```python
from build123d import *

# Parameters (mm, degrees)
EXTRUDE_1_DEPTH     = 13
EXTRUDE_2_DEPTH     = 3
EXTRUDE_3_DEPTH     = 1
CUT_EXTRUDE_1_DEPTH = 16
SKETCH_5_W          = 2
SKETCH_5_H          = 5
EXTRUDE_4_DEPTH     = 15
FILLET_1_R          = 2
SKETCH_6_W          = 1.000000004
SKETCH_6_H          = 5
SKETCH_6_W_2        = 0.999999996
SKETCH_6_W_3        = 1
EXTRUDE_5_DEPTH     = 9
SKETCH_7_W          = 2.859887346
SKETCH_7_H          = 6.332607693
SKETCH_7_W_2        = 2.383674024
SKETCH_7_H_2        = 6.268510199
SKETCH_7_W_3        = 2.540472095
SKETCH_7_H_3        = 6.351983774
EXTRUDE_7_DEPTH     = 1.5
SKETCH_8_R          = 1.317694444
CUT_EXTRUDE_2_DEPTH = 21.5
SKETCH_9_R          = 1.323361973
CUT_EXTRUDE_3_DEPTH = 3.5
FILLET_2_R          = 2
SKETCH_10_R         = 2
CUT_EXTRUDE_4_DEPTH = 3.5
SKETCH_11_R         = 2
CUT_EXTRUDE_5_DEPTH = 3.5
CHAMFER_1_SIZE      = 1


with BuildPart() as part:
    # Эскиз1 → Бобышка-Вытянуть1 (new body)
    with BuildSketch(Plane.XY):
        with BuildLine():
            Line((-24.03751348, 4.570186882), (-3.03751348, 4.570186882))
            ThreePointArc((-3.03751348, 4.570186882), (-0.916193137, 3.691507225), (-0.03751348, 1.570186882))
            Line((-0.03751348, 1.570186882), (-0.03751348, -9.429813118))
            Line((-0.03751348, -9.429813118), (-5.53751348, -14.429813118))
            Line((-5.53751348, -14.429813118), (-21.53751348, -14.429813118))
            Line((-21.53751348, -14.429813118), (-27.03751348, -9.429813118))
            Line((-27.03751348, -9.429813118), (-27.03751348, 1.570186882))
            ThreePointArc((-27.03751348, 1.570186882), (-26.158833824, 3.691507225), (-24.03751348, 4.570186882))
        make_face()
    extrude(amount=EXTRUDE_1_DEPTH)

    # Эскиз2 → Бобышка-Вытянуть2 (add)
    with BuildSketch(Plane.XY.offset(13)):
        with BuildLine():
            Line((-24.253629022, 6.070186882), (-2.821397929, 6.070186882))
            ThreePointArc((-2.821397929, 6.070186882), (-1.598940451, 5.87880838), (-0.493459013, 5.322985739))
            Line((-0.493459013, 5.322985739), (9.290425441, -1.679071989))
            ThreePointArc((9.290425441, -1.679071989), (10.962486488, -4.932373697), (9.289607579, -8.185254927))
            Line((9.289607579, -8.185254927), (-0.493722264, -15.183197119))
            ThreePointArc((-0.493722264, -15.183197119), (-1.598864627, -15.738588249), (-2.820843349, -15.929813118))
            Line((-2.820843349, -15.929813118), (-24.254183602, -15.929813118))
            ThreePointArc((-24.254183602, -15.929813118), (-25.476162332, -15.738588247), (-26.5813047, -15.183197109))
            Line((-26.5813047, -15.183197109), (-36.364634505, -8.185254887))
            ThreePointArc((-36.364634505, -8.185254887), (-38.037513448, -4.932373739), (-36.365452436, -1.679072079))
            Line((-36.365452436, -1.679072079), (-26.581567951, 5.322985729))
            ThreePointArc((-26.581567951, 5.322985729), (-25.476086508, 5.878808377), (-24.253629022, 6.070186882))
        make_face()
    extrude(amount=EXTRUDE_2_DEPTH)

    # Эскиз3 → Бобышка-Вытянуть3 (add)
    with BuildSketch(Plane.XY.offset(16)):
        with BuildLine():
            Line((-24.254183602, -15.929813118), (-2.820843349, -15.929813118))
            ThreePointArc((-2.820843349, -15.929813118), (0.007639796, -14.758184221), (1.179156647, -11.929654667))
            Line((1.179156647, -11.929654667), (1.178602071, 2.070186882))
            ThreePointArc((1.178602071, 2.070186882), (0.007029196, 4.898614007), (-2.821397929, 6.070186882))
            Line((-2.821397929, 6.070186882), (-24.253629022, 6.070186882))
            ThreePointArc((-24.253629022, 6.070186882), (-27.082056147, 4.898614007), (-28.253629022, 2.070186882))
            Line((-28.253629022, 2.070186882), (-28.254183602, -11.929813118))
            ThreePointArc((-28.254183602, -11.929813118), (-27.082610727, -14.758240243), (-24.254183602, -15.929813118))
        make_face()
    extrude(amount=EXTRUDE_3_DEPTH)

    # Эскиз4 → Вырез-Вытянуть1 (cut)
    with BuildSketch(Plane.XY.offset(17)):
        with BuildLine():
            Line((-24.537513476, 3.070186882), (-2.537513476, 3.070186882))
            ThreePointArc((-2.537513476, 3.070186882), (-1.476853304, 2.630847054), (-1.037513476, 1.570186882))
            Line((-1.037513476, 1.570186882), (-1.037513476, -8.208875847))
            ThreePointArc((-1.037513476, -8.208875847), (-1.185558621, -8.858658943), (-1.600470904, -9.380179061))
            Line((-1.600470904, -9.380179061), (-5.626642493, -12.601116332))
            ThreePointArc((-5.626642493, -12.601116332), (-6.067174653, -12.845255597), (-6.563685065, -12.929813118))
            Line((-6.563685065, -12.929813118), (-20.511341887, -12.929813118))
            ThreePointArc((-20.511341887, -12.929813118), (-21.007852299, -12.845255597), (-21.448384458, -12.601116332))
            Line((-21.448384458, -12.601116332), (-25.474556047, -9.380179061))
            ThreePointArc((-25.474556047, -9.380179061), (-25.88946833, -8.858658943), (-26.037513476, -8.208875847))
            Line((-26.037513476, -8.208875847), (-26.037513476, 1.570186882))
            ThreePointArc((-26.037513476, 1.570186882), (-25.598173647, 2.630847054), (-24.537513476, 3.070186882))
        make_face()
    extrude(amount=-CUT_EXTRUDE_1_DEPTH, mode=Mode.SUBTRACT)

    # Эскиз5 → Бобышка-Вытянуть4 (add)
    with BuildSketch(Plane.XY.offset(1)):
        with Locations((-21.537513476, -1.775325657)):
            Rectangle(SKETCH_5_W, SKETCH_5_H)
        with Locations((-13.537513476, -6.926056238)):
            Rectangle(SKETCH_5_W, SKETCH_5_H)
        with Locations((-5.537513476, -1.775325657)):
            Rectangle(SKETCH_5_W, SKETCH_5_H)
    extrude(amount=EXTRUDE_4_DEPTH)

    # Скругление1
    fillet_1_edges = [part.edges().sort_by_distance(p)[0] for p in [
        (-21.537513476, -4.275325657, 16),
        (-21.537513476, 0.724674343, 16),
        (-13.537513476, -9.426056238, 16),
        (-13.537513476, -4.426056238, 16),
        (-5.537513476, -4.275325657, 16),
        (-5.537513476, 0.724674343, 16),
    ]]
    fillet(fillet_1_edges, radius=FILLET_1_R)

    # Эскиз6 → Бобышка-Вытянуть5 (add)
    with BuildSketch(Plane(origin=(0, 0, 0), x_dir=(-1, 0, 0), z_dir=(0, 0, -1))):
        with Locations((5.037513478, -1.775325657)):
            Rectangle(SKETCH_6_W, SKETCH_6_H)
        with Locations((22.037513478, -1.775325657)):
            Rectangle(SKETCH_6_W_2, SKETCH_6_H)
        with Locations((13.628958145, -6.926056238)):
            Rectangle(SKETCH_6_W_3, SKETCH_6_H)
    extrude(amount=EXTRUDE_5_DEPTH)

    # Эскиз7 → Бобышка-Вытянуть7 (add)
    with BuildSketch(Plane(origin=(0, 0, 0), x_dir=(-1, 0, 0), z_dir=(0, 0, -1))):
        with Locations((5.059990277, -1.840113397)):
            Rectangle(SKETCH_7_W, SKETCH_7_H)
        with Locations((13.656892737, -6.928034415)):
            Rectangle(SKETCH_7_W_2, SKETCH_7_H_2)
        with Locations((22.046734018, -1.830425356)):
            Rectangle(SKETCH_7_W_3, SKETCH_7_H_3)
    extrude(amount=EXTRUDE_7_DEPTH)

    # Эскиз8 → Вырез-Вытянуть2 (cut)
    with BuildSketch(Plane(origin=(-4.537513476, 0, 0), x_dir=(0, 0, -1), z_dir=(1, 0, 0))):
        with Locations((6.23718035, -1.561929148)):
            Circle(SKETCH_8_R)
    extrude(amount=-CUT_EXTRUDE_2_DEPTH, mode=Mode.SUBTRACT)

    # Эскиз9 → Вырез-Вытянуть3 (cut)
    with BuildSketch(Plane(origin=(-13.128958145, 0, 0), x_dir=(0, 0, -1), z_dir=(1, 0, 0))):
        with Locations((6.266853337, -6.932739708)):
            Circle(SKETCH_9_R)
    extrude(amount=-CUT_EXTRUDE_3_DEPTH, mode=Mode.SUBTRACT)

    # Скругление2
    fillet_2_edges = [part.edges().sort_by_distance(p)[0] for p in [
        (-5.037513478, -4.275325657, -9),
        (-5.037513478, 0.724674343, -9),
        (-22.037513478, 0.724674343, -9),
        (-22.037513478, -4.275325657, -9),
        (-13.628958145, -9.426056238, -9),
        (-13.628958145, -4.426056238, -9),
    ]]
    fillet(fillet_2_edges, radius=FILLET_2_R)

    # Эскиз10 → Вырез-Вытянуть4 (cut)
    with BuildSketch(Plane.XY.offset(16)):
        with Locations((6.462486524, -4.931870875)):
            Circle(SKETCH_10_R)
    extrude(amount=-CUT_EXTRUDE_4_DEPTH, mode=Mode.SUBTRACT)

    # Эскиз11 → Вырез-Вытянуть5 (cut)
    with BuildSketch(Plane.XY.offset(16)):
        with Locations((-33.537513476, -4.931870875)):
            Circle(SKETCH_11_R)
    extrude(amount=-CUT_EXTRUDE_5_DEPTH, mode=Mode.SUBTRACT)

    # Фаска1
    chamfer_1_edges = [part.edges().sort_by_distance(p)[0] for p in [
        (4.462486524, -4.931870875, 16),
        (-35.537513476, -4.931870875, 16),
    ]]
    chamfer(chamfer_1_edges, length=CHAMFER_1_SIZE)


solid = part.part
```
Can you work these out from the model? Positions are in its coordinate system, mm. A direction names the side the tool comes from. Coordinates: 2 decimals unless noted, no trailing zeros. Write each loop counter-clockwise with the first axis right and the second up, starting at its lowest first coordinate (ties: lowest second). Pieces come first, ordered by that corner, then holes. Notation, with made-up numbers: (15, 89.25) - (56, 89.25) arc R22 ccw to (56, 127.25) - close; hole circle Ø11 at (-3, 44). An arc over 180 degrees is marked (long way). Return JSON: item names as keys, results as strings.
Q1. If we section it at C-C (x = -8): Please give me the cut outline in (y, z).
Computed values:
{"outline": "(-15.93, 13) - (-14.43, 13) - (-14.43, 0) - (4.57, 0) - (4.57, 13) - (6.07, 13) - (6.07, 17) - (3.07, 17) - (3.07, 1) - (-12.93, 1) - (-12.93, 17) - (-15.93, 17) - close"}
Q2. If we section it at A-A (z = 11.5): Count the separate pieces of the cut face and the enclosed holes in it, then the cut area to 3 significant figures.
Computed values:
{"separate pieces": "4", "enclosed holes": "1", "area": "133 mm2"}
Q3. If we section it at D-D (z = -5.5): Please give me the cut outline in (x, y).
Computed values:
{"outline": "(-22.54, -4.28) - (-21.54, -4.28) - (-21.54, -2.65) - (-22.54, -2.65) - close; (-22.54, -0.47) - (-21.54, -0.47) - (-21.54, 0.72) - (-22.54, 0.72) - close; (-14.13, -9.43) - (-13.13, -9.43) - (-13.13, -8.01) - (-14.13, -8.01) - close; (-14.13, -5.85) - (-13.13, -5.85) - (-13.13, -4.43) - (-14.13, -4.43) - close; (-5.54, -4.28) - (-4.54, -4.28) - (-4.54, -2.65) - (-5.54, -2.65) - close; (-5.54, -0.47) - (-4.54, -0.47) - (-4.54, 0.72) - (-5.54, 0.72) - close"}
Q4. Please list where these lines run through material, in increasing order: L1, parallel to X at y = -4.5, z = -1.25; L2, parallel to X at y = 0.5, z = -0.25; L3, parallel to X at y = -2.25, z = 10. Write a range as from..to.
Computed values:
{"L1": "x = -23.32..-20.78, -14.85..-12.47, -6.49..-3.63", "L2": "x = -23.32..-20.78, -6.49..-3.63", "L3": "x = -27.04..-26.04, -22.54..-20.54, -6.54..-4.54, -1.04..-0.04"}
Q5. I'm going to push flat-ended pins straight in: pin 1 Ø3 at (x, z) = (-15, 1.5) entering from -Y; pin 2 Ø10 at (y, z) = (-5, 1.5) entering from +X; pin 3 Ø1.6 at (x, z) = (-5.5, 4.5) entering from +Y. Where does each tip first touch, or does it pass through?
Computed values:
{"pin 1": "stops at y = -14.43", "pin 2": "stops at x = -0.04", "pin 3": "stops at y = 4.57"}
Q6. On a 3-axis mill with a long thin cutter (end or side, diameter ignored), from which of +Z, -Z, +X, -X, +Y, -Y can I reach the whole of each face in a straight line? I mean faces 4 (the flat face through (-13, -15, 13)), 5 (the flat face through (-22, -5.006, -1)), 6 (the cylindrical face through (-21.524, -3.705, 15.399)), 7 (the flat face through (-5.538, -2, -4)). Say none if no direction works.
Computed values:
{"face 4": "-Z", "face 5": "-Z, -X, -Y", "face 6": "+Z", "face 7": "-Z, +Y, -Y"}
Q7. Thinking about a two-plate mould opening in Y: for faces 1 (the flat face through (-31.542, 1.773, 14.479)), 2 (the flat face through (-4.538, -2, -4)), 3 (the flat face through (-22, -4.275, 7)), which applies, +Y half, -Y half, draft (parallel to the pull), parting line (faces both ways), or undercut?
Computed values:
{"face 1": "+Y half", "face 2": "draft", "face 3": "undercut"}
Q8. If we section it at B-B (z = -0.5): Please give me the cut outline in (x, y).
Computed values:
{"outline": "(-23.32, -5.01) - (-20.78, -5.01) - (-20.78, 1.35) - (-23.32, 1.35) - close; (-14.85, -10.06) - (-12.47, -10.06) - (-12.47, -3.79) - (-14.85, -3.79) - close; (-6.49, -5.01) - (-3.63, -5.01) - (-3.63, 1.33) - (-6.49, 1.33) - close"}
